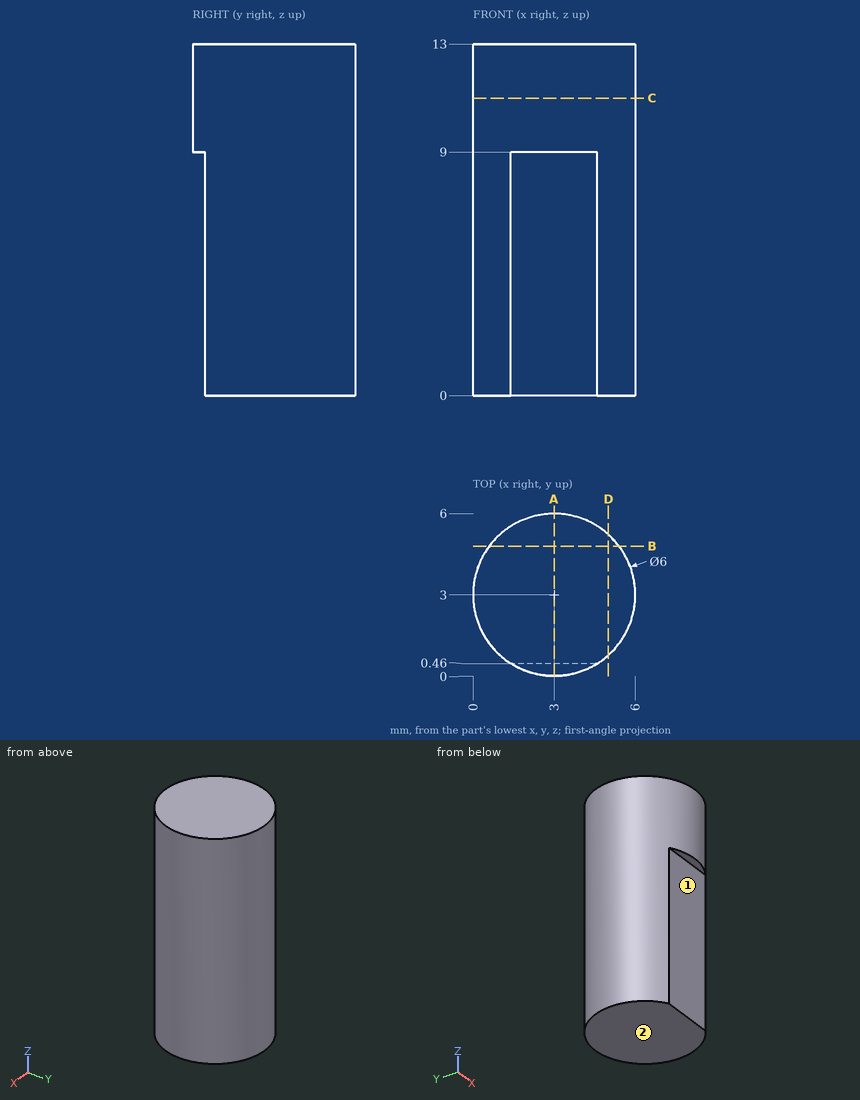
Print and shaded views of the part. All mm, measured from the part's lowest x, y and z. A direction names the side the tool comes from. Give positions to 0.01 mm unless a question says otherwise; leave off trailing zeros. Loops run counter-clockwise (first coordinate to the right, second up) from the corner with the lowest first, then second, coordinate; pieces in that order, holes last.
1) Flat gauge pins, fed straight in: pin 1 Ø1 at (x, z) = (1.5, 10) entering from +Y; pin 2 Ø1 at (y, z) = (5, 7) entering from +X; pin 3 Ø1.6 at (x, z) = (3, 6) entering from -Y. Where does each tip first touch, or does it go through?
2) Saw through at A-A (x = 3). Write the cut outline in (y, z).
3) Saw through at B-B (y = 4.8). Write the cut outline in (x, z), plus the area to 3 significant figures.
4) Saw through at C-C (z = 11). Write the cut outline in (x, y).
5) Wall check: line 1 (Y direction, x = 3.15, z = 6); line 2 (Y direction, x = 1.3, z = 8); line 3 (X direction, y = 0.8, z = 6). Give the ranges that are in metal, low to high.
6) Tool access for the marked faces 1 and 2: list every direction of +Z, -Z, +X, -X, +Y, -Y with a clear straight run to the whole face (end or side of a thin tool).
7) Saw through at D-D (x = 5). Write the cut outline in (y, z), plus the area to 3 significant figures.
Answer block:
1. pin 1: stops at y = 5.83
1. pin 2: stops at x = 5.6
1. pin 3: stops at y = 0.46
2. outline: (0, 9) - (0.46, 9) - (0.46, 0) - (6, 0) - (6, 13) - (0, 13) - close
3. outline: (0.6, 0) - (5.4, 0) - (5.4, 13) - (0.6, 13) - close
3. area: 62.4 mm2
4. outline: circle Ø6 at (3, 3)
5. line 1: y = 0.46 to 6
5. line 2: y = 0.53 to 5.47
5. line 3: x = 0.96 to 5.04
6. face 1: -Z, +X, -X, -Y
6. face 2: -Z, +X, -X, +Y, -Y
7. outline: (0.76, 0) - (5.24, 0) - (5.24, 13) - (0.76, 13) - close
7. area: 58.1 mm2
